Check sheet for the modelled part. Datum: model origin and axes. Units: mm. A direction names the side the tool comes from. Round coordinates to 2 decimals unless told otherwise and drop trailing zeros. Order: outer loops, then holes, each group sorted by start corner. A loop starts at its lowest first (then second) coordinate and runs counter-clockwise, first axis right, second up. Notation, with made-up numbers: M 65,-7.75 L 85,-7.75 A22 cw 85,27.25 Z; hole C -38,46.25 d9. An arc over 180 degrees is marked long. One line per item, written item: value. Start each with the question number.
(1) Depth check by flat-ended pin: pin 1 Ø3 at (x, z) = (-39, 1) entering from +Y; pin 2 Ø1.5 at (y, z) = (-31.5, 2) entering from +X; pin 3 Ø4 at (x, y) = (-38.5, 3.5) entering from +Z. Enter the tip coordinate at first touch or a pass-through.
(2) Access from +Z, -Z, +X, -X, +Y, -Y to the whole of each face (thin tool, end or side, straight path). Record for faces 5 (the face through (38, -29.9, 1)), 6 (the face through (-37, 0, 2.8)), 7 (the face through (-38, -29.9, 1)), 8 (the face through (17.6, -2, 3)).
(3) Cross-section at A-A, the plane y = 35. Enter the section's corners in (x, z), and give its area (3 significant figures).
(4) Cross-section at D-D, the plane x = 1. Enter the section's corners in (y, z), and give its area (3 significant figures).
(5) Release check for a two-part mould opening along Y. For faces 1 (the face through (-17, -22.03, 2.46)), 2 (the face through (-38, 29.9, 1)), 3 (the face through (37, 0, 2.8)), 4 (the face through (17.03, -22, 2.46)) record: released by +Y, released by -Y, zero draft, split by the parting line, or undercut.
(6) Cross-section at C-C, the plane y = -27. Enter the section's corners in (x, z).
(7) Thickness scan on L1, parallel to X at y = -35, z = 3.5; L2, parallel to Y at x = 29.9, z = 2.75; L3, parallel to Y at x = -14, z = 4.65. Record the ranges inside material, lowest first.
(8) Cross-section at B-B, the plane z = 2. Count the separate pieces of the cut face and the enclosed holes in it, and give its area (3 significant figures).
Autodesk Inventor part; units mm, degrees
ref_plane "YZ Plane" through (0, 0, 0) normal (1, 0, 0) x (0, 1, 0)
ref_plane "XZ Plane" through (0, 0, 0) normal (0, 1, 0) x (-1, 0, 0)
ref_plane "XY Plane" through (0, 0, 0) normal (0, 0, 1) x (1, 0, 0)
sketch "スケッチ1" plane through (0, 0, 0) normal (0, 0, 1) x (1, 0, 0)
  circle A0 centre (0, 0) radius 27.6
  line L0 (-40, 40) -> (40, 40)
  line L1 (40, 40) -> (40, -40)
  line L2 (40, -40) -> (-40, -40)
  line L3 (-40, -40) -> (-40, 40)
  dimension "d0" = 55.2
  dimension "d1" = 40
  dimension "d2" = 80
  dimension "d3" = 80
  dimension "d4" = 40
extrude "押し出し1" add sketch "スケッチ1" along normal blind 5 contours A0 | L0 L1 L2 L3
sketch "スケッチ3" plane through (0, 0, 5) normal (0, 0, 1) x (1, 0, 0)
  line L0 (40, -40) -> (-40, -40)
  line L1 (-40, 40) -> (-34.9, 40)
  line L2 (-34.9, 40) -> (-34.9, -40)
  line L3 (-34.9, -40) -> (-40, -40)
  line L4 (-40, -40) -> (-40, 40)
  line L5 (40, 40) -> (34.9, 40)
  line L6 (34.9, 40) -> (34.9, -40)
  line L7 (34.9, -40) -> (40, -40)
  line L8 (40, -40) -> (40, 40)
  dimension "d17" = 5.1
  dimension "d18" = 5.1
extrude "押し出し3" cut sketch "スケッチ3" against normal blind 2.2
sketch "スケッチ4" plane through (0, 0, 0) normal (0, 0, -1) x (-1, 0, 0)
  line L0 (-40, 40) -> (-34.9, 40)
  line L1 (-34.9, 40) -> (-34.9, 29.9)
  line L2 (-34.9, 29.9) -> (-40, 29.9)
  line L3 (-40, 29.9) -> (-40, 40)
  line L4 (-40, -40) -> (-34.9, -40)
  line L5 (-34.9, -40) -> (-34.9, -29.9)
  line L6 (-34.9, -29.9) -> (-40, -29.9)
  line L7 (-40, -29.9) -> (-40, -40)
  line L8 (40, 40) -> (34.9, 40)
  line L9 (34.9, 40) -> (34.9, 29.9)
  line L10 (34.9, 29.9) -> (40, 29.9)
  line L11 (40, 29.9) -> (40, 40)
  line L12 (40, -40) -> (34.9, -40)
  line L13 (34.9, -40) -> (34.9, -29.9)
  line L14 (34.9, -29.9) -> (40, -29.9)
  line L15 (40, -29.9) -> (40, -40)
  dimension "d21" = 5.1
  dimension "d22" = 10.1
  dimension "d23" = 10.1
  dimension "d24" = 10.1
  dimension "d25" = 5.1
  dimension "d26" = 5.1
  dimension "d27" = 5.1
  dimension "d28" = 10.1
extrude "押し出し4" cut sketch "スケッチ4" against normal through all
sketch "スケッチ5" plane through (0, 0, 0) normal (0, 0, -1) x (-1, 0, 0)
  line L0 (-40, -29.9) -> (-34.9, -29.9)
  line L1 (-34.9, -29.9) -> (-34.9, -40)
  line L2 (34.9, -40) -> (34.9, -29.9)
  line L3 (34.9, -29.9) -> (40, -29.9)
  line L4 (40, 29.9) -> (34.9, 29.9)
  line L5 (34.9, 29.9) -> (34.9, 40)
  line L6 (-34.9, 40) -> (-34.9, 29.9)
  line L7 (-34.9, 29.9) -> (-40, 29.9)
  point P0 (-35.9, 29.9)
  point P1 (-35.9, -29.9)
  point P2 (35.9, -29.9)
  point P3 (35.9, 29.9)
  dimension "d31" = 1
  dimension "d32" = 1
  dimension "d33" = 1
  dimension "d34" = 1
hole "Hole1" at (35.9, 29.9, 0) at (35.9, -29.9, 0) at (-35.9, -29.9, 0) at (-35.9, 29.9, 0) direction (0, 0, 1) diameter 2 end through all
sketch "スケッチ6" plane through (0, 0, 5) normal (0, 0, 1) x (1, 0, 0)
  line L0 (-17.6, 17.6) -> (17.6, 17.6)
  line L1 (17.6, 17.6) -> (17.6, -17.6)
  line L2 (17.6, -17.6) -> (-17.6, -17.6)
  line L3 (-17.6, -17.6) -> (-17.6, 17.6)
  line L4 (-17.6, -17.6) -> (17.6, -17.6)
  line L5 (17.6, -17.6) -> (17.6, -22.6)
  line L6 (17.6, -22.6) -> (-17.6, -22.6)
  line L7 (-17.6, -22.6) -> (-17.6, -17.6)
  point P0 (0, 0)
  dimension "d42" = 35.2
  dimension "d43" = 35.2
  dimension "d44" = 17.6
  dimension "d45" = 17.6
  dimension "d46" = 5
extrude "押し出し5" cut sketch "スケッチ6" against normal through all
fillet "フィレット1" radius 2 4 edges at (-17.6, 17.6, 2.5) (-17.6, -22.6, 2.5) (17.6, -22.6, 2.5) (17.6, 17.6, 2.5)
sketch "スケッチ7" plane through (0, 0, 5) normal (0, 0, 1) x (1, 0, 0)
  line L0 (-34.9, 40) -> (-34.9, -40)
  line L1 (34.9, -40) -> (-34.9, -40)
  line L2 (34.9, -40) -> (34.9, 40)
  line L3 (-34.9, 40) -> (34.9, 40)
  point P0 (0, 0)
  point P1 (-29.9, 35)
  point P2 (-29.9, -35)
  point P3 (29.9, -35)
  point P4 (29.9, 35)
  dimension "d50" = 5
  dimension "d51" = 5
  dimension "d52" = 5
  dimension "d53" = 5
  dimension "d54" = 5
  dimension "d55" = 5
  dimension "d56" = 5
  dimension "d57" = 5
hole "Hole2" at (-29.9, 35, 5) at (-29.9, -35, 5) at (29.9, -35, 5) at (29.9, 35, 5) direction (0, 0, -1) diameter 3 end through all
sketch "スケッチ8" plane through (0, 0, 5) normal (0, 0, 1) x (1, 0, 0)
  line L0 (15.6, -22.6) -> (-15.6, -22.6)
  line L1 (-5, -22.6) -> (5, -22.6)
  line L2 (5, -22.6) -> (5, -32.6)
  line L3 (5, -32.6) -> (-5, -32.6)
  line L4 (-5, -32.6) -> (-5, -22.6)
  point P0 (0, 0)
  dimension "d65" = 10
  dimension "d66" = 5
  dimension "d67" = 10
extrude "押し出し6" cut sketch "スケッチ8" against normal through all
fillet "フィレット2" radius 2 2 edges at (-5, -32.6, 2.5) (5, -32.6, 2.5)
equation "\"d1\" = 0.5 * d2"
equation "\"d3\" = d2"
equation "\"d18\" = d17"
equation "\"d23\" = d22"
equation "\"d25\" = d21"
equation "\"d26\" = d21"
equation "\"d27\" = d21"
equation "\"d28\" = d22"
properties part number "JointA1"
Values found:
1. pin 1: y = 29.9
1. pin 2: x = 34.9
1. pin 3: z = 2.8
2. face 5: +Z, -Z, +X, -Y
2. face 6: +Z, -X, +Y, -Y
2. face 7: +Z, -Z, -X, -Y
2. face 8: +Z, -Z
3. outline: M -34.9,0 L -31.4,0 L -31.4,5 L -34.9,5 Z; M -28.4,0 L 28.4,0 L 28.4,5 L -28.4,5 Z; M 31.4,0 L 34.9,0 L 34.9,5 L 31.4,5 Z
3. area: 319 mm^2
4. outline: M -40,0 L -32.6,0 L -32.6,5 L -40,5 Z; M 17.6,0 L 40,0 L 40,5 L 17.6,5 Z
4. area: 149 mm^2
5. face 1: undercut
5. face 2: released by +Y
5. face 3: zero draft
5. face 4: undercut
6. outline: M -40,0 L -5,0 L -5,5 L -34.9,5 L -34.9,2.8 L -40,2.8 Z; M 5,0 L 40,0 L 40,2.8 L 34.9,2.8 L 34.9,5 L 5,5 Z
7. L1: -34.9 to -31.4, -28.4 to 28.4, 31.4 to 34.9
7. L2: -40 to -36.5, -33.5 to 33.5, 36.5 to 40
7. L3: -40 to -22.6, 17.6 to 40
8. separate pieces: 1
8. enclosed holes: 5
8. area: 4,650 mm^2
